For this review, take the finished solid that the model builds, in its own axes (mm). Face numbers are marked on the shaded views. A direction names the side the tool comes from. Give positions to 0.01 mm unless a question says otherwise; leave off trailing zeros. Write each loop counter-clockwise with the first axis right and the second up, starting at its lowest first coordinate (ties: lowest second). Pieces come first, ordered by that corner, then holes.
Q1. We need section A-A (x = -62). Write out the cut boundary in (y, z), then the cut area to 3 significant figures.
Q2. Mouldability with a two-part tool opening along X and no side actions: class the marked faces 4, 5 and 6 as released by +X, released by -X, zero draft, split by the parting line, or undercut.
Q3. We need section B-B (z = -20). Write out the cut boundary in (x, y), then the cut area to 4 significant figures.
Q4. We need section C-C (y = 1). Write out the cut boundary in (x, z) (1 decimal).
Q5. For line 1 (X direction, y = 5.25, z = -24.5); line 2 (Z direction, x = -86.5, y = 9.75); line 3 (X direction, y = 10, z = -10), list the stretches that pass through material, from the lowest coordinate up.
Q6. Insertion check: P1, Ø2, axis at x = -82.5, y = 4.5, coming from the +Z side; P2, Ø0.9, axis at x = -129.5, y = 5.5, coming from the -Z side; P3, Ø6, axis at x = -56.5, y = 6.5, coming from the +Z side. Each pin has a flat end and moves straight along its axis. Give the tip position at first contact, or say it passes through.
Q7. Machinability: for the marked faces 1, 2 and 3, which of the approach directions +Z, -Z, +X, -X, +Y, -Y give a long, thin tool a straight path to every point of the face, cutting with its end or side? Answer none if there is none.
Q8. We need section D-D (x = -84). Write out the cut boundary in (y, z).
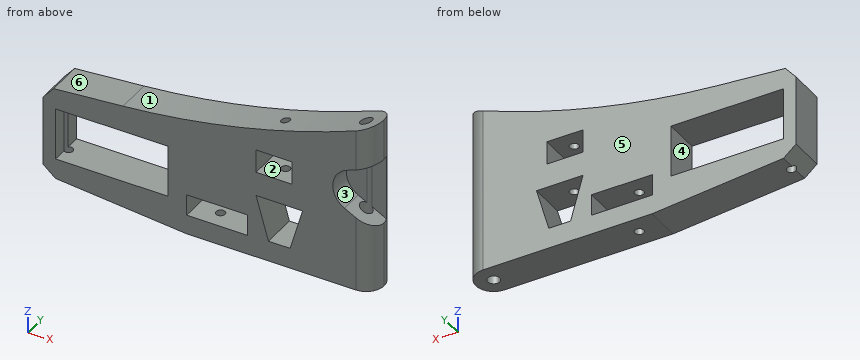
```python
from build123d import *

# Parameters (mm, degrees)
SKETCH1_W                = 36.8554
SKETCH1_H                = 17.1196
SKETCH1_W_2              = 19.8882
SKETCH1_H_2              = 6.985
SKETCH1_W_3              = 11.8237
SKETCH1_H_3              = 7.62
BOSS_EXTRUDE1_DEPTH      = 11.684
CUT_EXTRUDE7_DEPTH       = 139.474144195
CUT_EXTRUDE7_DEPTH_BACK  = 139.474144195
SKETCH3_R                = 1.4605
CUT_EXTRUDE8_DEPTH       = 139.474144228
SKETCH4_R                = 1.4605
CUT_EXTRUDE9_DEPTH       = 18.034
SKETCH5_R                = 1.4605
CUT_EXTRUDE10_DEPTH      = 16.3195
CUT_EXTRUDE11_DEPTH      = 139.474144228
CUT_EXTRUDE11_DEPTH_BACK = 139.474144228
SKETCH6_R                = 1.9685
CUT_EXTRUDE12_DEPTH      = 7.62


with BuildPart() as part:
    # Sketch1 → Boss-Extrude1 (new body)
    with BuildSketch(Plane(origin=(0, 0, 0), x_dir=(1, 0, 0), z_dir=(0, 1, 0))):
        with BuildLine():
            Line((-25.4, 34.376681198), (-67.6656, 34.376681198))
            Line((-67.6656, 34.376681198), (-86.5378, 34.376681198))
            Line((-86.5378, 34.376681198), (-129.54, 30.312681198))
            Line((-129.54, 30.312681198), (-133.6294, 26.832881198))
            Line((-133.6294, 26.832881198), (-133.6294, 3.896681198))
            Line((-133.6294, 3.896681198), (-130.1496, -0.192718802))
            Line((-130.1496, -0.192718802), (-107.423789895, -2.069465817))
            ThreePointArc((-107.423789895, -2.069465817), (-65.592867309, -8.938068561), (-25.4, -22.411642903))
            Line((-25.4, -22.411642903), (-25.4, 34.376681198))
        make_face()
        with Locations((-111.1123, 15.098081198)):
            Rectangle(SKETCH1_W, SKETCH1_H, mode=Mode.SUBTRACT)
        with Locations((-76.64751862, 24.508781198)):
            Rectangle(SKETCH1_W_2, SKETCH1_H_2, mode=Mode.SUBTRACT)
        with Locations((-57.99455, 1.650285214)):
            Rectangle(SKETCH1_W_3, SKETCH1_H_3, mode=Mode.SUBTRACT)
        Polygon((-63.9064, 13.384739375), (-48.6664, 13.384739375), (-52.7304, 27.608739375), (-59.8424, 27.608739375), align=None, mode=Mode.SUBTRACT)
    extrude(amount=BOSS_EXTRUDE1_DEPTH)

    # Sketch2 → Cut-Extrude7 (cut, two sides: drawn at the far end of the back side and taken through both)
    with BuildSketch(Plane.XY.offset(-CUT_EXTRUDE7_DEPTH_BACK)):
        with BuildLine():
            Line((-25.4, 11.684), (-31.242, 11.684))
            ThreePointArc((-31.242, 11.684), (-27.111082184, 9.972917816), (-25.4, 5.842))
            Line((-25.4, 5.842), (-25.4, 11.684))
        make_face()
        with BuildLine():
            Line((-25.4, 0), (-25.4, 5.842))
            ThreePointArc((-25.4, 5.842), (-27.111082184, 1.711082184), (-31.242, 0))
            Line((-31.242, 0), (-25.4, 0))
        make_face()
    extrude(amount=CUT_EXTRUDE7_DEPTH + CUT_EXTRUDE7_DEPTH_BACK, mode=Mode.SUBTRACT)

    # Sketch3 → Cut-Extrude8 (cut, through all)
    with BuildSketch(Plane.XY):
        with Locations((-128.6891, 5.842)):
            Circle(SKETCH3_R)
    extrude(amount=-CUT_EXTRUDE8_DEPTH, mode=Mode.SUBTRACT)

    # Sketch4 → Cut-Extrude9 (cut)
    with BuildSketch(Plane(origin=(0, 0, -34.376681198), x_dir=(-1, 0, 0), z_dir=(0, 0, -1))):
        with Locations((78.9178, 5.842)):
            Circle(SKETCH4_R)
    extrude(amount=-CUT_EXTRUDE9_DEPTH, mode=Mode.SUBTRACT)

    # Sketch5 → Cut-Extrude10 (cut, symmetric)
    with BuildSketch(Plane.XY):
        with Locations((-57.6326, 5.842)):
            Circle(SKETCH5_R)
    extrude(amount=CUT_EXTRUDE10_DEPTH, both=True, mode=Mode.SUBTRACT)

    # Sketch6 → Cut-Extrude11 (cut, two sides: drawn at the far end of the back side and taken through both)
    with BuildSketch(Plane.XY.offset(-CUT_EXTRUDE11_DEPTH_BACK)):
        with Locations((-31.242, 5.842)):
            Circle(SKETCH6_R)
    extrude(amount=CUT_EXTRUDE11_DEPTH + CUT_EXTRUDE11_DEPTH_BACK, mode=Mode.SUBTRACT)

    # Sketch8 → Cut-Extrude12 (cut)
    with BuildSketch(Plane.XZ):
        with BuildLine():
            Line((-34.127459258, 5.550738999), (-23.258487089, 9.749460917))
            Line((-23.258487089, 9.749460917), (-23.258487089, -12.81023225))
            Line((-23.258487089, -12.81023225), (-23.258487089, -13.936212277))
            Line((-23.258487089, -13.936212277), (-34.934853819, -7.703267827))
            ThreePointArc((-34.934853819, -7.703267827), (-38.784988232, -0.817133676), (-34.127459258, 5.550738999))
        make_face()
    extrude(amount=-CUT_EXTRUDE12_DEPTH, mode=Mode.SUBTRACT)


solid = part.part
```
Computed:
1. outline: (0, -34.38) - (11.68, -34.38) - (11.68, -20.06) - (0, -20.06) - close; (0, -13.38) - (11.68, -13.38) - (11.68, -5.46) - (0, -5.46) - close; (0, 2.16) - (11.68, 2.16) - (11.68, 9.86) - (0, 9.86) - close
1. area: 350 mm2
2. face 4: undercut
2. face 5: zero draft
2. face 6: released by -X
3. outline: (-133.63, 0) - (-129.54, 0) - (-129.54, 4.65) arc R1.46 cw to (-129.54, 7.03) - (-129.54, 11.68) - (-133.63, 11.68) - close; (-92.68, 0) - (-62.02, 0) - (-62.02, 11.68) - (-92.68, 11.68) - close; (-50.56, 0) - (-31.24, 0) arc R5.84 ccw to (-31.24, 11.68) - (-50.56, 11.68) - close; hole circle Ø2.92 at (-78.92, 5.84); hole circle Ø3.94 at (-31.24, 5.84)
3. area: 665.5 mm2
4. outline: (-133.6, -26.8) - (-129.5, -30.3) - (-86.5, -34.4) - (-28, -34.4) - (-28, -11.4) - (-34.9, -7.7) arc R7.3 cw to (-34.1, 5.6) - (-28, 7.9) - (-28, 21.3) arc R264.1 cw to (-107.4, 2.1) - (-130.1, 0.2) - (-133.6, -3.9) - close; hole (-129.5, -23.7) - (-92.7, -23.7) - (-92.7, -6.5) - (-129.5, -6.5) - close; hole (-86.6, -28) - (-66.7, -28) - (-66.7, -21) - (-86.6, -21) - close; hole (-63.9, -13.4) - (-59.8, -27.6) - (-52.7, -27.6) - (-48.7, -13.4) - close; hole (-63.9, -5.5) - (-52.1, -5.5) - (-52.1, 2.2) - (-63.9, 2.2) - close
5. line 1: x = -133.63 to -130.02, -127.35 to -86.59, -66.7 to -60.73, -51.84 to -33.12, -29.36 to -25.43
5. line 2: z = -34.38 to -28, -21.02 to 4.64
5. line 3: x = -133.63 to -129.54, -92.68 to -27.14
6. P1: stops at z = 5.51
6. P2: stops at z = 0
6. P3: stops at z = 12.24
7. face 1: +Z, -X, +Y, -Y
7. face 2: +Y, -Y
7. face 3: +X, -Y
8. outline: (0, -34.38) - (11.68, -34.38) - (11.68, -28) - (0, -28) - close; (0, -21.02) - (11.68, -21.02) - (11.68, 5.06) - (0, 5.06) - close
